Design review of the part built by this model. Coordinates are the model's own, in mm. A direction names the side the tool comes from. Round coordinates to 2 decimals unless told otherwise and drop trailing zeros. Order: outer loops, then holes, each group sorted by start corner. A loop starts at its lowest first (then second) coordinate and runs counter-clockwise, first axis right, second up. Notation, with made-up numbers: (52, 67) - (61, 67) arc R15 cw to (61, 91) - close; hole circle Ø4 at (13.25, 26). An arc over 180 degrees is marked (long way). Write item = value, one per line.
from build123d import *

# Parameters (mm, degrees)
EXTRU_MINCE1_DEPTH         = 2.3
CONG_1_R                   = 2.3
ESQUISSE2_W                = 40
ESQUISSE2_H                = 49.6
BOSS_EXTRU_1_DEPTH         = 2.3
R_P_TITION_LIN_AIRE1_COUNT = 2
R_P_TITION_LIN_AIRE1_PITCH = 40
CONG_2_R                   = 2.3
ESQUISSE3_R                = 9
BOSS_EXTRU_2_DEPTH         = 25
BOSS_EXTRU_2_DRAFT         = -2


with BuildPart() as part:
    # Esquisse1 → Extru.-Mince1 (new, symmetric)
    with BuildSketch(Plane.XY):
        Polygon((-4.3, -57), (-4.3, -47.3), (2.3, -47.3), (2.3, 2.3), (-8.9, 2.3), (-8.9, -12), (-4.3, -12), (-4.3, -2.3), (-2.3, -2.3), (-2.3, -42.7), (-8.9, -42.7), (-8.9, -57), align=None)
    extru_mince1 = extrude(amount=EXTRU_MINCE1_DEPTH, both=True)

    # Congé1
    cong_1_edges = [part.edges().sort_by_distance(p)[0] for p in [
        (-6.6, -57, -2.3),
        (-4.3, -52.15, -2.3),
        (-1, -47.3, -2.3),
        (2.3, -22.5, -2.3),
        (-3.3, 2.3, -2.3),
        (-8.9, -4.85, -2.3),
        (-6.6, -12, -2.3),
        (-4.3, -7.15, -2.3),
        (-3.3, -2.3, -2.3),
        (-2.3, -22.5, -2.3),
        (-5.6, -42.7, -2.3),
        (-8.9, -49.85, -2.3),
        (-5.6, -42.7, 2.3),
        (-2.3, -22.5, 2.3),
        (-3.3, -2.3, 2.3),
        (-4.3, -7.15, 2.3),
        (-6.6, -12, 2.3),
        (-8.9, -4.85, 2.3),
        (-3.3, 2.3, 2.3),
        (2.3, -22.5, 2.3),
        (-1, -47.3, 2.3),
        (-4.3, -52.15, 2.3),
        (-6.6, -57, 2.3),
        (-8.9, -49.85, 2.3),
    ]]
    fillet(cong_1_edges, radius=CONG_1_R - 0.0001)  # a hair under: the kernel refuses the full size

    # Esquisse2 → Boss.-Extru.1 (add)
    with BuildSketch(Plane(origin=(0, 0, 0), x_dir=(0, 0, -1), z_dir=(1, 0, 0))):
        with Locations((-20, -22.5)):
            Rectangle(ESQUISSE2_W, ESQUISSE2_H)
    extrude(amount=BOSS_EXTRU_1_DEPTH)

    # Répétition linéaire1: Extru.-Mince1 ×2
    with Locations(*[(0, 0, i * R_P_TITION_LIN_AIRE1_PITCH) for i in range(1, R_P_TITION_LIN_AIRE1_COUNT)]):
        add(extru_mince1)

    # Congé2
    cong_2_edges = [part.edges().sort_by_distance(p)[0] for p in [
        (-5.6, -42.7, 42.3),
        (-2.3, -22.5, 42.3),
        (-3.3, -2.3, 42.3),
        (-4.3, -7.15, 42.3),
        (-6.6, -12, 42.3),
        (-8.9, -4.85, 42.3),
        (-3.3, 2.3, 42.3),
        (2.3, -22.5, 42.3),
        (-1, -47.3, 42.3),
        (-4.3, -52.15, 42.3),
        (-6.6, -57, 42.3),
        (-8.9, -49.85, 42.3),
        (-2.15, -47.3, 37.7),
        (-4.3, -52.15, 37.7),
        (-6.6, -57, 37.7),
        (-8.9, -49.85, 37.7),
        (-5.6, -42.7, 37.7),
        (-2.3, -22.5, 37.7),
        (-3.3, -2.3, 37.7),
        (-4.3, -7.15, 37.7),
        (-6.6, -12, 37.7),
        (-8.9, -4.85, 37.7),
        (-4.45, 2.3, 37.7),
    ]]
    fillet(cong_2_edges, radius=CONG_2_R - 0.0001)  # a hair under: the kernel refuses the full size


with BuildPart() as boss_extru_2_tool:
    # Esquisse3 → Boss.-Extru.2 (with draft: the straight prism first)
    with BuildSketch(Plane(origin=(2.3, 0, 0), x_dir=(0, 0, -1), z_dir=(1, 0, 0))):
        with Locations((-20, -17.3)):
            Circle(ESQUISSE3_R)
    extrude(amount=BOSS_EXTRU_2_DEPTH)
    # Boss.-Extru.2: the draft: its side faces are tilted about the plane it starts from
    boss_extru_2_sides = [boss_extru_2_tool.faces().sort_by_distance(p)[0] for p in [
        (14.8, -17.3, 29),
    ]]
    draft(boss_extru_2_sides, Plane(origin=(2.3, 0, 0), x_dir=(0, 0, -1), z_dir=(1, 0, 0)), BOSS_EXTRU_2_DRAFT)


with BuildPart() as part_1:
    add(part.part)

    # Boss.-Extru.2: add boss_extru_2_tool
    add(boss_extru_2_tool.part)


solid = part_1.part
Item 1: The part is to be moulded in two halves that separate along Z. For faces 1 (the face through (27.3, -17, 20)), 2 (the face through (-3.38, 1.64, -1.61)), 3 (the face through (-3.25, -1.34, 1.87)), 4 (the face through (-1.64, -22.81, 41.61)), say which applies: +Z half, -Z half, draft (parallel to the pull), parting line (faces both ways), or undercut.
Data:
face_1 = draft
face_2 = -Z half
face_3 = undercut
face_4 = +Z half
Item 2: Take a section at D-D, the plane x = 17. State the section outline as (y, z) points, and give its area (3 significant figures).
Data:
outline = circle Ø19.03 at (-17.3, 20)
area = 284 mm2
Item 3: Take a section at A-A, the plane y = -4. Count the separate pieces of the cut face and the enclosed holes in it, and give its area (3 significant figures).
Data:
separate_pieces = 3
enclosed_holes = 0
area = 150 mm2
Item 4: Insertion check: P1, Ø5.5, axis at x = -2, y = -41, coming from the +Z side; P2, Ø2, axis at x = 2.5, y = -5.5, coming from the +Z side; P3, Ø3, axis at y = -48.5, z = 11, coming from the -X side; P4, Ø6, axis at x = 0.5, z = 12, coming from the -Y side. Each pin has a flat end and moves straight along its axis. Give the tip position at first contact, or say it passes through.
Data:
P1 = 42.3
P2 = 41.74
P3 = 0
P4 = -47.3
Item 5: For faces 5 (the face through (-8.24, -4.95, 38.39)), 6 (the face through (-4.96, -5.92, 41.61)), 7 (the face through (-1.64, -22.81, 1.61)), 8 (the face through (1, -47.3, 20)), 9 (the face through (-6.568, -11.598, 38.702)), list the 3-axis set-ups (+Z, -Z, +X, -X, +Y, -Y) from which the entire face can be reached by the end or side of a thin tool; tool diameter is ignored.
Data:
face_5 = -X, +Y, -Y
face_6 = +Z
face_7 = none
face_8 = +Z, -Z, +X, -Y
face_9 = -X
Item 6: For line 1 along X through (y, z) = (-7, 9.5); line 2 along Z through (x, y) = (-1.5, -13); line 3 along Y through (x, z) = (1, 20.5), list the stretches that pass through material, from the lowest coordinate up. Write a range as [from, to].
Data:
line_1 = [0, 2.3]
line_2 = [-1.74, 1.74], [38.26, 41.74]
line_3 = [-47.3, 2.3]
Item 7: Take a section at B-B, the plane z = 20. State the section outline as (x, y) points.
Data:
outline = (0, -47.3) - (2.3, -47.3) - (2.3, -26.3) - (27.3, -27.17) - (27.3, -7.43) - (2.3, -8.3) - (2.3, 2.3) - (0, 2.3) - close
